Build history of the part. All positions in model axes, mm. Face numbers are marked on the shaded views. A direction names the side the tool comes from. Give positions to 0.01 mm unless a question says otherwise; leave off trailing zeros. Order: outer loops, then holes, each group sorted by start corner. A loop starts at its lowest first (then second) coordinate and runs counter-clockwise, first axis right, second up. Notation, with made-up numbers: M 62,0 L 77,0 A27 ccw 77,39 Z; hole C -3.5,88 d3. An arc over 180 degrees is marked long. One line per item, written item: value. Start each with the question number.
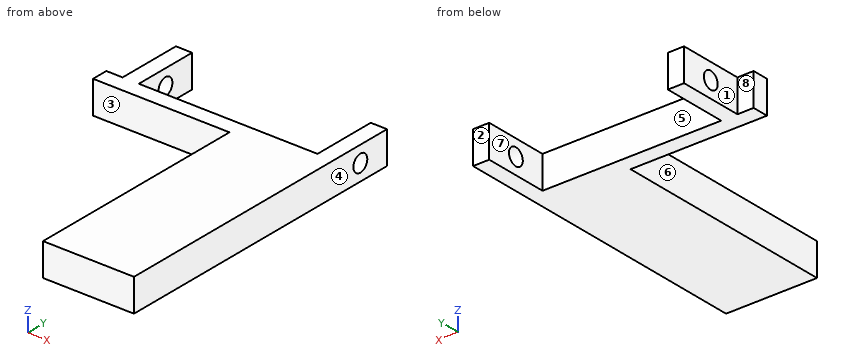
from build123d import *

# Parameters (mm, degrees)
EXTRUDE_1_DEPTH     = 10
SKETCH_3_R          = 2.6
CUT_EXTRUDE_1_DEPTH = 116.542200083


with BuildPart() as part:
    # ｽｹｯﾁ2 → ﾎﾞｽ - 押し出し1 (new body)
    with BuildSketch(Plane.XY):
        Polygon((-60, 75), (-5, 75), (-5, 95), (0, 95), (0, 75), (0, 70), (0, 0), (-28, 0), (-28, 70), (-70, 70), (-70, 75), (-65, 75), (-65, 95), (-60, 95), align=None)
    extrude(amount=EXTRUDE_1_DEPTH)

    # ｽｹｯﾁ3 → ｶｯﾄ - 押し出し1 (cut, through all)
    with BuildSketch(Plane.ZY.offset(65)):
        with Locations((5, 85)):
            Circle(SKETCH_3_R)
    extrude(amount=-CUT_EXTRUDE_1_DEPTH, mode=Mode.SUBTRACT)


solid = part.part
1) Slice it at A-A (z = 5). List the corners of the cut face in (x, y), plus the area to 3 significant figures.
2) Slice it at B-B (y = 81). List the corners of the cut face in (x, z), plus the area to 3 significant figures.
3) Slice it at C-C (x = -54.5). List the corners of the cut face in (y, z).
4) Tool access for the marked faces 1, 2, 3, 4 and 5: list every direction of +Z, -Z, +X, -X, +Y, -Y with a clear straight run to the whole face (end or side of a thin tool).
5) Drop flat-ended pins along their axis: P1, Ø2, axis at x = -52.5, z = 7, coming from the -Y side; P2, Ø3, axis at x = -37, z = 4.5, coming from the +Y side; P3, Ø5, axis at y = 81.5, z = 5.5, coming from the -X side. Give the stop position or say it passes through.
6) Pull direction X, two halves, no side cores. Call the marked faces 6, 7 and 8: pulls with the +X half, pulls with the -X half, needs draft (parallel to the pull), parting line crosses it, or undercut.
7) Drill centre lines: line 1 (X direction, y = 80, z = 5.25); line 2 (Y direction, x = -63, z = 5); line 3 (Y direction, x = -2.6, z = 5). Where is each one in solid material? Low to high.
8) Slice it at D-D (y = 50). List the corners of the cut face in (x, z).
Results list:
1. outline: M -70,70 L -28,70 L -28,0 L 0,0 L 0,82.4 L -5,82.4 L -5,75 L -60,75 L -60,82.4 L -65,82.4 L -65,75 L -70,75 Z; M -65,87.6 L -60,87.6 L -60,95 L -65,95 Z; M -5,87.6 L 0,87.6 L 0,95 L -5,95 Z
1. area: 2,460 mm²
2. outline: M -65,0 L -60,0 L -60,10 L -65,10 Z; M -5,0 L 0,0 L 0,10 L -5,10 Z
2. area: 100 mm²
3. outline: M 70,0 L 75,0 L 75,10 L 70,10 Z
4. face 1: +Z, -Z, -X, +Y
4. face 2: +Z, -Z, +X, -X, +Y
4. face 3: +Z, -Z, -X, -Y
4. face 4: +Z, -Z, +X, +Y, -Y
4. face 5: +Z, -Z, +Y
5. P1: stops at y = 70
5. P2: stops at y = 75
5. P3: stops at x = -65
6. face 6: pulls with the -X half
6. face 7: undercut
6. face 8: needs draft
7. line 1: x = -65 to -60, -5 to 0
7. line 2: y = 70 to 82.4, 87.6 to 95
7. line 3: y = 0 to 82.4, 87.6 to 95
8. outline: M -28,0 L 0,0 L 0,10 L -28,10 Z
